from build123d import *

# Parameters (mm, degrees)
F0_W        = 59
F0_H        = 15
F0_R        = 0.75
F0_R_2      = 1.25
F0_R_3      = 2.35
F0_R_4      = 0.875
F1_DEPTH    = 1
F2_W        = 0.5
F2_H        = 4
F3_DEPTH    = 3
F4_T4_DEPTH = 16.4300979278
F4_T9_DEPTH = 16.4300979278


# Not quite as in the source:
# - a fillet or chamfer that OpenCascade refuses, or shapes differently, is made with other operations: its cross-section is extruded or revolved along the edge and cut away or added


with BuildPart() as f1:
    # F0 (on Top) → F1 (new body)
    with BuildSketch(Plane.XY):
        with Locations((10, 12.3232733458)):
            Rectangle(F0_W, F0_H)
        with Locations((-3.81, 7.2432733458)):
            Circle(F0_R, mode=Mode.SUBTRACT)
        with Locations((3.81, 7.2432733458)):
            Circle(F0_R, mode=Mode.SUBTRACT)
        with Locations((-5.08, 12.3232733458)):
            Circle(F0_R_2, mode=Mode.SUBTRACT)
        with Locations((0, 12.3232733458)):
            Circle(F0_R_3, mode=Mode.SUBTRACT)
        with Locations((5.08, 12.3232733458)):
            Circle(F0_R_2, mode=Mode.SUBTRACT)
        with Locations((16.19, 7.2432733458)):
            Circle(F0_R, mode=Mode.SUBTRACT)
        with Locations((23.81, 7.2432733458)):
            Circle(F0_R, mode=Mode.SUBTRACT)
        with Locations((14.92, 12.3232733458)):
            Circle(F0_R_2, mode=Mode.SUBTRACT)
        with Locations((20, 12.3232733458)):
            Circle(F0_R_3, mode=Mode.SUBTRACT)
        with BuildLine():
            ThreePointArc((-16.3, 14.5025628582), (-14.5, 16.3025628582), (-12.7, 14.5025628582))
            Line((-12.7, 14.5025628582), (-12.7, 10.5025628582))
            ThreePointArc((-12.7, 10.5025628582), (-14.5, 8.7025628582), (-16.3, 10.5025628582))
            Line((-16.3, 10.5025628582), (-16.3, 14.5025628582))
        make_face(mode=Mode.SUBTRACT)
        with Locations((-3.81, 14.8632733458)):
            Circle(F0_R_4, mode=Mode.SUBTRACT)
        with Locations((2.54, 17.4032733458)):
            Circle(F0_R_4, mode=Mode.SUBTRACT)
        with Locations((16.19, 14.8632733458)):
            Circle(F0_R_4, mode=Mode.SUBTRACT)
        with Locations((25.08, 12.3232733458)):
            Circle(F0_R_2, mode=Mode.SUBTRACT)
        with BuildLine():
            ThreePointArc((36.3, 10.5025628582), (34.5, 8.7025628582), (32.7, 10.5025628582))
            Line((32.7, 10.5025628582), (32.7, 14.5025628582))
            ThreePointArc((32.7, 14.5025628582), (34.5, 16.3025628582), (36.3, 14.5025628582))
            Line((36.3, 14.5025628582), (36.3, 10.5025628582))
        make_face(mode=Mode.SUBTRACT)
        with Locations((22.54, 17.4032733458)):
            Circle(F0_R_4, mode=Mode.SUBTRACT)
    extrude(amount=F1_DEPTH)

    # F2 (on face) → F3 (join)
    with BuildSketch(Plane.XY.offset(1)):
        Polygon((39.5, 19.8232733458), (-19.5, 19.8232733458), (-19.5, 18.8232733458), (9.5, 18.8232733458), (10.5, 18.8232733458), (39.5, 18.8232733458), align=None)
        Polygon((9.5, 5.8232733458), (-19.5, 5.8232733458), (-19.5, 4.8232733458), (39.5, 4.8232733458), (39.5, 5.8232733458), (10.5, 5.8232733458), (10, 5.8232733458), align=None)
        with Locations((10.25, 7.8232733458)):
            Rectangle(F2_W, F2_H)
        Polygon((10.5, 18.8232733458), (9.5, 18.8232733458), (9.5, 14.8232733458), (10, 14.8232733458), (10.5, 14.8232733458), align=None)
        with Locations((9.75, 7.8232733458)):
            Rectangle(F2_W, F2_H)
    extrude(amount=-F3_DEPTH)

    # F4: chamfer of 3 on 2 edges, made by hand


with BuildPart() as f4_tool2:
    # F4_s3 → F4_t4 (new body)
    with BuildSketch(Plane.YZ.offset(18.2150489639)):
        Polygon((9.8232733458, 1), (6.8232733458, -2), (9.8232733458, -2), align=None)
    extrude(amount=-F4_T4_DEPTH)

    split(bisect_by=Plane.XY, keep=Keep.BOTTOM)


with BuildPart() as f1_1:
    add(f1.part)

    # F4_t1: cut F4_tool2
    add(f4_tool2.part, mode=Mode.SUBTRACT)


with BuildPart() as f4_tool7:
    # F4_s8 → F4_t9 (new body)
    with BuildSketch(Plane.YZ.offset(1.7849510361)):
        Polygon((14.8232733458, 1), (17.8232733458, -2), (14.8232733458, -2), align=None)
    extrude(amount=F4_T9_DEPTH)

    split(bisect_by=Plane.XY, keep=Keep.BOTTOM)


with BuildPart() as f1_2:
    add(f1_1.part)

    # F4_t6: cut F4_tool7
    add(f4_tool7.part, mode=Mode.SUBTRACT)


solid = f1_2.part
Geometry: final body of the model. Coordinates: model frame, mm. A direction names the side the tool comes from. Give positions to 0.01 mm unless a question says otherwise; leave off trailing zeros. Loops run counter-clockwise (first coordinate to the right, second up) from the corner with the lowest first, then second, coordinate; pieces in that order, holes last. Notation, with made-up numbers: (57, 57.5) -> (82, 57.5) arc R30 ccw to (82, 91.5) -> close; hole circle Ø9 at (39, 58.5). An arc over 180 degrees is marked (long way). Put each result on its own line as item: value.
1. Ray query, line 1 along Y through (x, z) = (5.08, 0.55); line 2 along X through (y, z) = (7.5, 0.6); line 3 along Y through (x, z) = (22.54, 0.5). Return the intervals inside material, ascending. Write a range as [from, to].
Taken from the geometry:
line 1: y = [4.82, 11.07], [13.57, 19.82]
line 2: x = [-19.5, -4.51], [-3.11, 3.11], [4.51, 15.49], [16.89, 23.11], [24.51, 39.5]
line 3: y = [4.82, 16.53], [18.28, 19.82]
2. Set-up query: faces 5 (the flat face through (10, 12, 0)), 6 (the flat face through (-16.3, 12.5, 0.5)), 7 (the flat face through (10.5, 7, -1)), 8 (the flat face through (-5, 18.823, -1)). Return all of +Z, -Z, +X, -X, +Y, -Y with unobstructed straight access to the full face (end or side cutting, diameter ignored); none if empty.
Taken from the geometry:
face 5: -Z
face 6: +Z, -Z
face 7: -Z, +X
face 8: -Z, -X
3. Cut plane C-C (x = -10). Return the cut outline in (y, z), plus the area to 3 significant figures.
Taken from the geometry:
outline: (4.82, -2) -> (5.82, -2) -> (5.82, 0) -> (18.82, 0) -> (18.82, -2) -> (19.82, -2) -> (19.82, 1) -> (4.82, 1) -> close
area: 19.0 mm2
4. Cut plane D-D (x = 20). Return the cut outline in (y, z), plus the area to 3 significant figures.
Taken from the geometry:
outline: (4.82, -2) -> (5.82, -2) -> (5.82, 0) -> (9.97, 0) -> (9.97, 1) -> (4.82, 1) -> close; (14.67, 0) -> (18.82, 0) -> (18.82, -2) -> (19.82, -2) -> (19.82, 1) -> (14.67, 1) -> close
area: 14.3 mm2
5. Cut plane B-B (z = -1.15). Return the cut outline in (x, y).
Taken from the geometry:
outline: (-19.5, 4.82) -> (39.5, 4.82) -> (39.5, 5.82) -> (10.5, 5.82) -> (10.5, 7.67) -> (9.5, 7.67) -> (9.5, 5.82) -> (-19.5, 5.82) -> close; (-19.5, 18.82) -> (9.5, 18.82) -> (9.5, 16.97) -> (10.5, 16.97) -> (10.5, 18.82) -> (39.5, 18.82) -> (39.5, 19.82) -> (-19.5, 19.82) -> close
6. Pin query (flat end, axial travel): P1, Ø2, axis at x = -3.81, y = 14.86, coming from the -Z side; P2, Ø1.6, axis at x = 2.54, y = 17.4, coming from the +Z side; P3, Ø1.7, axis at x = 16.19, y = 7.24, coming from the +Z side; P4, Ø1, axis at y = 8, z = -1, coming from the +X side. Return the tip coordinate at first contact, or that it passes through.
Taken from the geometry:
P1: stops at z = 0
P2: passes through
P3: stops at z = 1
P4: stops at x = 10.5
7. Cut plane A-A (x = 5.08). Return the cut outline in (y, z).
Taken from the geometry:
outline: (4.82, -2) -> (5.82, -2) -> (5.82, 0) -> (11.07, 0) -> (11.07, 1) -> (4.82, 1) -> close; (13.57, 0) -> (18.82, 0) -> (18.82, -2) -> (19.82, -2) -> (19.82, 1) -> (13.57, 1) -> close
8. Pull-direction query (Y, two-part tool) for faces 1 (the flat face through (32.7, 12.5, 0.5)), 2 (the cylindrical face through (-14.46, 8.703, 0.493)), 3 (the flat face through (10, 5, -2)), 4 (the flat face through (10, 4.823, -1)); classes: released by +Y, released by -Y, zero draft, split by the parting line, or undercut.
Taken from the geometry:
face 1: undercut
face 2: undercut
face 3: zero draft
face 4: released by -Y
